```python
from build123d import *

# Parameters (mm, degrees)
F1_DEPTH = 72.9
F2_T     = -3


with BuildPart() as f1:
    # F0 (on Top) → F1 (new body)
    with BuildSketch(Plane.XY):
        Polygon((12.249669, 29.573318), (-12.249669, 29.573318), (-29.573318, 12.249669), (-29.573318, -12.249669), (-12.249669, -29.573318), (12.249669, -29.573318), (29.573318, -12.249669), (29.573318, 12.249669), align=None)
    extrude(amount=F1_DEPTH)

    # F2
    f2_openings = [f1.faces().sort_by_distance(p)[0] for p in [
        (0, 0, 72.9),
    ]]
    offset(amount=F2_T, openings=f2_openings)


solid = f1.part
```
Geometry check sheet. Reference: the model listing, model coordinates, mm. A direction names the side the tool comes from. Coordinates: 2 decimals unless noted, no trailing zeros. Loops run counter-clockwise (first coordinate to the right, second up) from the corner with the lowest first, then second, coordinate; pieces in that order, holes last.
Item 1: Thickness scan on line 1 (X direction, y = 9.5, z = 43.5); line 2 (Z direction, x = -3.5, y = 22.5). Record the ranges inside material, lowest first.
Item 2: Go/stop test with flat-tipped pins: pin 1 Ø1 at (x, z) = (14, 25) entering from -Y; pin 2 Ø6 at (x, y) = (21, 19) entering from -Z; pin 3 Ø12 at (y, z) = (19.5, 43) entering from -X; pin 4 Ø4 at (y, z) = (21, 13.5) entering from -X. Record where each tip stops, or that it passes through.
Item 3: Release check for a two-part mould opening along Y. For faces 3 (the face through (0, -26.573, 37)), 4 (the face through (20, -20, 72.9)), 5 (the face through (20.79, -21.033, 35.94)) record: released by +Y, released by -Y, zero draft, split by the parting line, or undercut.
Item 4: Sectioned sample at B-B, the plane x = 2. Record the boundary of the cut face in (y, z), then the cut area to 3 significant figures.
Item 5: Access from +Z, -Z, +X, -X, +Y, -Y to the whole of each face (thin tool, end or side, straight path). Record for faces 1 (the face through (0, 26.573, 37)), 2 (the face through (0, -29.573, 36)).
Item 6: Sectioned sample at A-A, the plane z = 25. Record the boundary of the cut face in (x, y), then the cut area to 3 significant figures.
Check result:
1. line 1: x = -29.57 to -26.57, 26.57 to 29.57
1. line 2: z = 0 to 3
2. pin 1: stops at y = -28.32
2. pin 2: stops at z = 0
2. pin 3: stops at x = -28.32
2. pin 4: stops at x = -22.82
3. face 3: undercut
3. face 4: zero draft
3. face 5: released by -Y
4. outline: (-29.57, 0) - (29.57, 0) - (29.57, 72.9) - (26.57, 72.9) - (26.57, 3) - (-26.57, 3) - (-26.57, 72.9) - (-29.57, 72.9) - close
4. area: 597 mm2
5. face 1: +Z
5. face 2: +Z, -Z, +X, -X, -Y
6. outline: (-29.57, -12.25) - (-12.25, -29.57) - (12.25, -29.57) - (29.57, -12.25) - (29.57, 12.25) - (12.25, 29.57) - (-12.25, 29.57) - (-29.57, 12.25) - close; hole (-26.57, -11.01) - (-11.01, -26.57) - (11.01, -26.57) - (26.57, -11.01) - (26.57, 11.01) - (11.01, 26.57) - (-11.01, 26.57) - (-26.57, 11.01) - close
6. area: 558 mm2
